The listing builds one solid part. Answer for the finished solid, in the listing's coordinates (mm). A direction names the side the tool comes from. Give positions to 0.01 mm unless a question says otherwise; leave off trailing zeros.
```python
from build123d import *

# Parameters (mm, degrees)
BOSS_EXTRUDE1_DEPTH         = 85.399999968
SKETCH2_R                   = 19.3
SKETCH2_R_2                 = 17.008
BOSS_EXTRUDE2_DEPTH         = 2.5
DRAFT1_ANGLE                = 15
DOME1_FACE_RADIUS           = 16.338127019
DOME1_HEIGHT                = 1
F_1_4_CLEARANCE_HOLE1_D     = 6.7564
F_1_4_CLEARANCE_HOLE1_DEPTH = 8
F_1_4_CLEARANCE_HOLE1_TIP   = 2.029827343
M2X0_4_TAPPED_HOLE1_D       = 1.6
M2X0_4_TAPPED_HOLE1_DEPTH   = 2
M2X0_4_TAPPED_HOLE1_TIP     = 0.480688495
M2X0_4_TAPPED_HOLE2_D       = 1.6
M2X0_4_TAPPED_HOLE2_DEPTH   = 3.2
M2X0_4_TAPPED_HOLE2_TIP     = 0.480688495
M2X0_4_TAPPED_HOLE3_D       = 1.6
M2X0_4_TAPPED_HOLE3_DEPTH   = 3.2
M2X0_4_TAPPED_HOLE3_TIP     = 0.480688495
M2X0_4_TAPPED_HOLE4_D       = 1.6
M2X0_4_TAPPED_HOLE4_DEPTH   = 3.2
M2X0_4_TAPPED_HOLE4_TIP     = 0.480688495


with BuildPart() as part:
    # Sketch1 → Boss-Extrude1 (new body)
    with BuildSketch(Plane.XY):
        Polygon((-25, 25.5), (-23, 27.5), (23, 27.5), (25, 25.5), (25, -28), (23, -30), (-21, -30), (-25, -26), align=None)
    extrude(amount=BOSS_EXTRUDE1_DEPTH)

    # Sketch2 → Boss-Extrude2 (add)
    with BuildSketch(Plane.XY.offset(85.399999968)):
        with Locations(Location((0, 0, 0), (0, 0, 180))):
            Circle(SKETCH2_R)
        Circle(SKETCH2_R_2, mode=Mode.SUBTRACT)
    extrude(amount=BOSS_EXTRUDE2_DEPTH)

    # Draft1
    draft1_faces = [part.faces().sort_by_distance(p)[0] for p in [
        (-17.008, 0, 86.649999968),
    ]]
    draft(draft1_faces, Plane.XY.offset(87.899999968), DRAFT1_ANGLE)

    # Dome1: a dome of height H over a round flat face of radius A is a cap of a sphere of radius (A * A + H * H) / (2 * H)
    dome1_r = (DOME1_FACE_RADIUS * DOME1_FACE_RADIUS + DOME1_HEIGHT * DOME1_HEIGHT) / (2 * DOME1_HEIGHT)
    dome1_base = Plane((0, 0, 85.399999968), z_dir=(0, 0, 1))
    with Locations(dome1_base.offset(DOME1_HEIGHT - dome1_r)):
        dome1_ball = Sphere(dome1_r, mode=Mode.PRIVATE)
    add(split(dome1_ball, bisect_by=dome1_base, keep=Keep.TOP, mode=Mode.PRIVATE))

    # 1/4 Clearance Hole1
    with Locations(Plane.XZ.offset(30)):
        with Locations((0, 67.899999968)):
            Hole(F_1_4_CLEARANCE_HOLE1_D / 2, depth=F_1_4_CLEARANCE_HOLE1_DEPTH)
            with Locations((0, 0, -(F_1_4_CLEARANCE_HOLE1_DEPTH + F_1_4_CLEARANCE_HOLE1_TIP / 2))):  # 118° drill point
                Cone(0, F_1_4_CLEARANCE_HOLE1_D / 2, F_1_4_CLEARANCE_HOLE1_TIP, mode=Mode.SUBTRACT)

    # M2x0.4 Tapped Hole1
    with Locations(Plane(origin=(0, -30, 0), x_dir=(-1, 0, 0), z_dir=(0, -1, 0))):
        with Locations((-8, -51.899999968), (8, -51.899999968), (-8, -22.899999968), (8, -22.899999968), (13.5, -47.699999968), (-13.5, -47.699999968), (-13.5, -14.699999968), (13.5, -14.699999968)):
            Hole(M2X0_4_TAPPED_HOLE1_D / 2, depth=M2X0_4_TAPPED_HOLE1_DEPTH)
            with Locations((0, 0, -(M2X0_4_TAPPED_HOLE1_DEPTH + M2X0_4_TAPPED_HOLE1_TIP / 2))):  # 118° drill point
                Cone(0, M2X0_4_TAPPED_HOLE1_D / 2, M2X0_4_TAPPED_HOLE1_TIP, mode=Mode.SUBTRACT)

    # M2x0.4 Tapped Hole2
    with Locations(Plane(origin=(25, 0, 0), x_dir=(0, 0, -1), z_dir=(1, 0, 0))):
        with Locations((-77.899999968, 10), (-77.899999968, -11), (-4.899999968, 10), (-29.599999968, -15.4)):
            Hole(M2X0_4_TAPPED_HOLE2_D / 2, depth=M2X0_4_TAPPED_HOLE2_DEPTH)
            with Locations((0, 0, -(M2X0_4_TAPPED_HOLE2_DEPTH + M2X0_4_TAPPED_HOLE2_TIP / 2))):  # 118° drill point
                Cone(0, M2X0_4_TAPPED_HOLE2_D / 2, M2X0_4_TAPPED_HOLE2_TIP, mode=Mode.SUBTRACT)

    # M2x0.4 Tapped Hole3
    with Locations(Plane(origin=(0, 27.5, 0), x_dir=(1, 0, 0), z_dir=(0, 1, 0))):
        with Locations((-5, -72.899999968), (15, -52.899999968), (-5, -52.899999968), (-10, -72.899999968), (10, -72.899999968), (10, -52.899999968), (-10, -52.899999968), (-10, -24.899999968), (10, -24.899999968)):
            Hole(M2X0_4_TAPPED_HOLE3_D / 2, depth=M2X0_4_TAPPED_HOLE3_DEPTH)
            with Locations((0, 0, -(M2X0_4_TAPPED_HOLE3_DEPTH + M2X0_4_TAPPED_HOLE3_TIP / 2))):  # 118° drill point
                Cone(0, M2X0_4_TAPPED_HOLE3_D / 2, M2X0_4_TAPPED_HOLE3_TIP, mode=Mode.SUBTRACT)

    # M2x0.4 Tapped Hole4
    with Locations(Plane.ZY.offset(25)):
        with Locations((2.699999968, 4.5), (2.699999968, -9.5)):
            Hole(M2X0_4_TAPPED_HOLE4_D / 2, depth=M2X0_4_TAPPED_HOLE4_DEPTH)
            with Locations((0, 0, -(M2X0_4_TAPPED_HOLE4_DEPTH + M2X0_4_TAPPED_HOLE4_TIP / 2))):  # 118° drill point
                Cone(0, M2X0_4_TAPPED_HOLE4_D / 2, M2X0_4_TAPPED_HOLE4_TIP, mode=Mode.SUBTRACT)


solid = part.part
```
1) Given P1, Ø5, axis at x = 10, y = -2, coming from the +Z side; P2, Ø1, axis at x = 15, z = 52.9, coming from the +Y side; P3, Ø1.3, axis at x = 10, z = 24.9, coming from the +Y side, each flat-ended and moving along its own axis, determine where each tip first touches the part or whether it passes through.
Geometry says:
P1: stops at z = 86.18
P2: stops at y = 24.12
P3: stops at y = 24.21
2) Straight lines are drawn through the part: probe 1 along Z at (x, y) = (23.1, 10); probe 2 along Z at (x, y) = (-5, 25.7); probe 3 along Y at (x, z) = (22, 78). For each, find the intervals that lie inside material, in ascending order.
Geometry says:
probe 1: z = 0 to 4.1, 5.7 to 77.1, 78.7 to 85.4
probe 2: z = 0 to 52.1, 53.7 to 72.1, 73.7 to 85.4
probe 3: y = -30 to -11.79, -10.21 to 9.21, 10.79 to 27.5
3) A tool of negligible diameter and unlimited length cuts with its end or side. For faces 1 (the cylindrical face through (0.44, -25.94, 71.25)), 2 (the flat face through (24, -29, 42)), 3 (the flat face through (0, -20, 85.4)), from which of +Z, -Z, +X, -X, +Y, -Y can it reach the whole face along a straight path? Write none if from no direction.
Geometry says:
face 1: -Y
face 2: +Z, -Z, +X, -Y
face 3: +Z
